CAD build for the part. Positions are in the model's coordinates, mm. A direction names the side the tool comes from. Give positions to 0.01 mm unless a question says otherwise; leave off trailing zeros. Write each loop counter-clockwise with the first axis right and the second up, starting at its lowest first coordinate (ties: lowest second). Pieces come first, ordered by that corner, then holes. Notation, with made-up numbers: (40, -40) -> (69, -40) arc R7 cw to (69, -28) -> close; hole circle Ø2 at (52.25, 5). An arc over 180 degrees is marked (long way). Use one line per item in the form item = value. Start each with the question number.
from build123d import *

# Parameters (mm, degrees)
RISER_DEPTH             = 7
SKETCH2_R               = 1.475
MOUNTING_HOLES_DEPTH    = 44.150898021
SKETCH3_W               = 40.15
SKETCH3_H               = 5.15
RECESS_DEPTH            = 2
FLANGE_DEPTH            = 7
SKETCH5_W               = 26.797240136
SKETCH5_H               = 6.925
FLANGE_CUTOUT_DEPTH     = 5
ANGLE_CUTOUT_DEPTH      = 44.886216515
ANGLE_CUTOUT_DEPTH_BACK = 44.886216515
FLANGE_CHAMFER_1_SIZE   = 1
FLANGE_CHAMFER_2_SIZE   = 1


with BuildPart() as part:
    # Sketch1 → Riser (new body)
    with BuildSketch(Plane(origin=(0, 0, 0), x_dir=(1, 0, 0), z_dir=(0, 1, 0))):
        Polygon((2.000418161, 7), (42, 7), (42, 0), (0, 0), (0, 5.75), align=None)
    extrude(amount=RISER_DEPTH)

    # Sketch2 → Mounting Holes (cut, through all)
    with BuildSketch(Plane.XZ):
        with Locations(Location((37, -3.5, 0), (0, 0, 270))):
            Circle(SKETCH2_R)
        with Locations(Location((5, -3.5, 0), (0, 0, 90))):
            Circle(SKETCH2_R)
    extrude(amount=-MOUNTING_HOLES_DEPTH, mode=Mode.SUBTRACT)

    # Sketch3 → Recess (cut)
    with BuildSketch(Plane(origin=(0, 7, 0), x_dir=(1, 0, 0), z_dir=(0, 1, 0))):
        with Locations((21, 3.5)):
            Rectangle(SKETCH3_W, SKETCH3_H)
    extrude(amount=-RECESS_DEPTH, mode=Mode.SUBTRACT)

    # Sketch4 → Flange (add)
    with BuildSketch(Plane(origin=(0, 0, 0), x_dir=(1, 0, 0), z_dir=(0, 1, 0))):
        Polygon((2.000418161, 7), (42, 7), (42, 14), (13.202759864, 14), align=None)
    extrude(amount=FLANGE_DEPTH)

    # Sketch5 → Flange Cutout (cut)
    with BuildSketch(Plane(origin=(0, 7, 0), x_dir=(1, 0, 0), z_dir=(0, 1, 0))):
        with Locations((27.601379932, 10.5375)):
            Rectangle(SKETCH5_W, SKETCH5_H)
        Polygon((2.120443251, 7.075), (13.202759864, 7.075), (13.202759864, 14), align=None)
    extrude(amount=-FLANGE_CUTOUT_DEPTH, mode=Mode.SUBTRACT)

    # Sketch7 → Angle Cutout (cut, two sides: drawn at the far end of the back side and taken through both)
    with BuildSketch(Plane.ZY.offset(-41).offset(-ANGLE_CUTOUT_DEPTH_BACK)):
        Polygon((-7.075, 7), (-14, 2), (-14, 7), align=None)
    extrude(amount=ANGLE_CUTOUT_DEPTH + ANGLE_CUTOUT_DEPTH_BACK, mode=Mode.SUBTRACT)

    # Flange Chamfer 1
    flange_chamfer_1_edges = [part.edges().sort_by_distance(p)[0] for p in [
        (27.601379932, 2, -7.075),
    ]]
    chamfer(flange_chamfer_1_edges, length=FLANGE_CHAMFER_1_SIZE)

    # Flange Chamfer 2
    flange_chamfer_2_edges = [part.edges().sort_by_distance(p)[0] for p in [
        (7.661601558, 2, -7.075),
    ]]
    chamfer(flange_chamfer_2_edges, length=FLANGE_CHAMFER_2_SIZE)


solid = part.part
1) Cut at D-D (y = 5.75). Give the cut face in (x, z) (3 decimals).
2) Cut at C-C (y = 1). Give the cut face in (x, z) (3 decimals).
3) 3-axis set-ups, long thin cutter, end or side, ignore diameter. For faces 1 (the face through (8, 5, -7.075)), 2 (the face through (41.507, 4.535, -10.489)), 3 (the face through (14.203, 3, -9)), 4 (the face through (21, 6, -0.925)): which of +Z, -Z, +X, -X, +Y, -Y reach the whole face in a straight line?
4) Pin check, flat tips, straight feed: pin 1 (8 mm diameter, centred on x = 4.5, z = -9, fed in from +Y); pin 2 (4 mm diameter, centred on y = 3.5, z = -10.5, fed in from -X); pin 3 (4 mm diameter, centred on x = 20.5, z = -4, fed in from +Y); pin 4 (6.5 mm diameter, centred on x = 8, z = -10.5, fed in from +Y) (3 decimals). Stop position of each tip, or through.
5) Two-plate mould, pull along Z, no slides. Class faces 5 (the face through (21, 6, -6.075)), 6 (the face through (0.925, 6, -3)), 7 (the face through (28, 1, -14)), 8 (the face through (11, 2, -10)): released by +Z, released by -Z, zero draft, split by the parting line, or undercut.
6) Cut at B-B (z = -3.5). Give the cut face in (x, y) (3 decimals).
7) Wall check: line 1 along X through (y, z) = (1.9, -3.5) (3 decimals); line 2 along X through (y, z) = (3.5, -8.75); line 3 along X through (y, z) = (6.5, -2.75) (3 decimals). Give the ranges that are in metal, low to high. Write a range as from..to.
8) Cut at A-A (x = 37). Give the cut face in (y, z) (3 decimals).
Final values:
q1.outline = (0, -5.75) -> (2.12, -7.075) -> (13.203, -7.075) -> (13.203, -8.806) -> (14.203, -8.806) -> (14.203, -7.075) -> (41, -7.075) -> (41, -8.806) -> (42, -8.806) -> (42, 0) -> (0, 0) -> close; hole (0.925, -6.075) -> (41.075, -6.075) -> (41.075, -0.925) -> (0.925, -0.925) -> close
q2.outline = (0, -5.75) -> (13.203, -14) -> (42, -14) -> (42, 0) -> (0, 0) -> close; hole circle Ø2.95 at (5, -3.5); hole circle Ø2.95 at (37, -3.5)
q3.face_1 = -Z, -X, +Y
q3.face_2 = -Z, +X, -X, +Y
q3.face_3 = -Z, +Y
q3.face_4 = +Y
q4.pin_1 = 7
q4.pin_2 = 5.48
q4.pin_3 = 5
q4.pin_4 = 2.825
q5.face_5 = undercut
q5.face_6 = undercut
q5.face_7 = released by -Z
q5.face_8 = zero draft
q6.outline = (0, 0) -> (3.525, 0) -> (3.525, 5) -> (0.925, 5) -> (0.925, 7) -> (0, 7) -> close; (6.475, 0) -> (35.525, 0) -> (35.525, 5) -> (6.475, 5) -> close; (38.475, 0) -> (42, 0) -> (42, 7) -> (41.075, 7) -> (41.075, 5) -> (38.475, 5) -> close
q7.line_1 = 0..3.525, 6.475..35.525, 38.475..42
q7.line_2 = 13.2..14.2, 41..42
q7.line_3 = 0..0.925, 41.075..42
q8.outline = (0, -14) -> (2, -14) -> (2, -8.075) -> (3, -7.075) -> (7, -7.075) -> (7, -6.075) -> (5, -6.075) -> (5, -4.975) -> (0, -4.975) -> close; (0, -2.025) -> (5, -2.025) -> (5, -0.925) -> (7, -0.925) -> (7, 0) -> (0, 0) -> close
